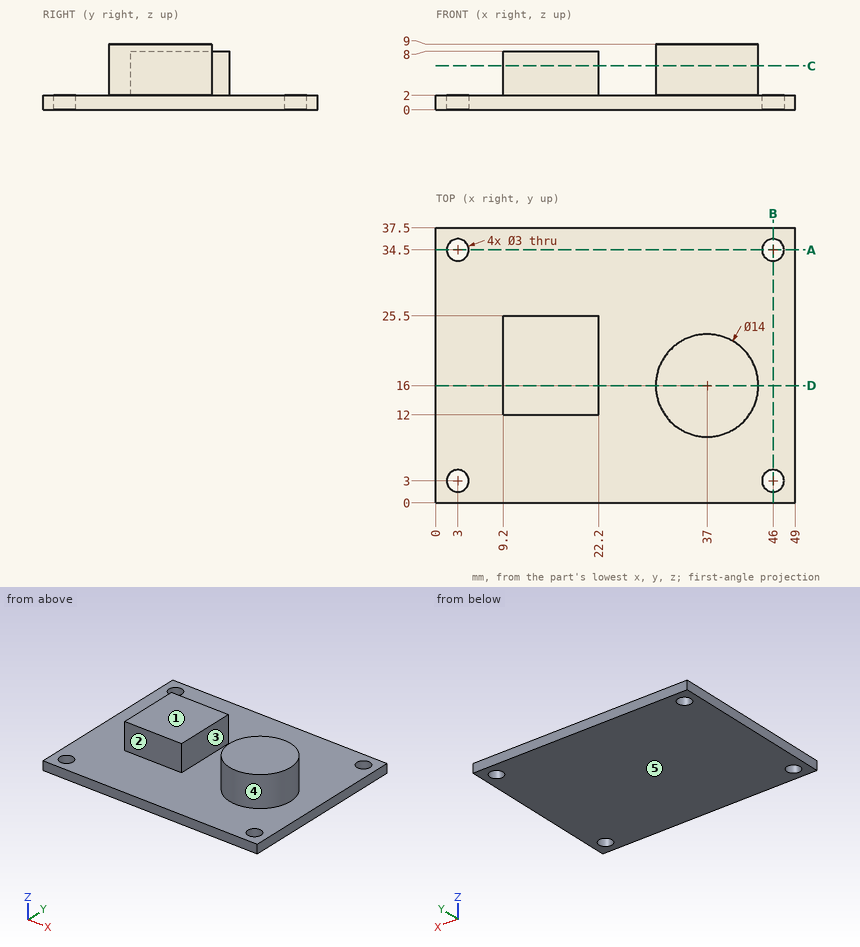
Can you work these out from the drawing? Everything is in mm from the part's minimum corner. A direction names the side the tool comes from. Coordinates: 2 decimals unless noted, no trailing zeros. Loops run counter-clockwise (first coordinate to the right, second up) from the corner with the lowest first, then second, coordinate; pieces in that order, holes last. Notation, with made-up numbers: M 7.5,14.25 L 60.5,14.25 A14 ccw 60.5,39.25 Z; hole C 2,71 d7. An arc over 180 degrees is marked long. Put each result on its own line as item: value. Start each with the question number.
(1) Thinking about a two-plate mould opening in X: for the marked faces 4 and 5, which applies, pulls with the +X half, pulls with the -X half, needs draft (parallel to the pull), parting line crosses it, or undercut?
(2) Will these pins go through, and if not, where does the flat tip stop? P1, Ø1.5, axis at x = 42.5, y = 10, coming from the +Z side; P2, Ø19, axis at x = 17, y = 16.5, coming from the +Z side; P3, Ø2, axis at y = 13.5, z = 3.5, coming from the +X side; P4, Ø1.8, axis at x = 3, y = 3, coming from the -Z side.
(3) For the marked faces 1, 2 and 3, which set-ups out of +Z, -Z, +X, -X, +Y, -Y let a thin tool reach every point of the face, with its end or its side?
(4) Suppose I cut it at C-C on z = 6. Please give me the cut outline in (x, y), then the cut area to 3 significant figures.
(5) Suppose I cut it at A-A on y = 34.5. Please give me the cut outline in (x, z), then the cut area to 3 significant figures.
(6) I need wall thicknesses on line 1 (Y direction, x = 46, z = 1.3); line 2 (Z direction, x = 33.5, y = 5); line 3 (Z direction, x = 12, y = 19.5). Which ranges of each line are inside material? Lowest first, please. Write a range as from..to.
(7) Suppose I cut it at D-D on y = 16. Please give me the cut outline in (x, z), then the cut area to 3 significant figures.
(8) Suppose I cut it at B-B on x = 46. Please give me the cut outline in (y, z), then the cut area to 3 significant figures.
Solutions:
1. face 4: undercut
1. face 5: needs draft
2. P1: stops at z = 2
2. P2: stops at z = 8
2. P3: stops at x = 43.84
2. P4: passes through
3. face 1: +Z, -X, +Y, -Y
3. face 2: +Z, -X, -Y
3. face 3: +Z, +Y, -Y
4. outline: M 9.2,12 L 22.2,12 L 22.2,25.5 L 9.2,25.5 Z; C 37,16 d14
4. area: 329 mm2
5. outline: M 0,0 L 1.5,0 L 1.5,2 L 0,2 Z; M 4.5,0 L 44.5,0 L 44.5,2 L 4.5,2 Z; M 47.5,0 L 49,0 L 49,2 L 47.5,2 Z
5. area: 86.0 mm2
6. line 1: y = 0..1.5, 4.5..33, 36..37.5
6. line 2: z = 0..2
6. line 3: z = 0..8
7. outline: M 0,0 L 49,0 L 49,2 L 44,2 L 44,9 L 30,9 L 30,2 L 22.2,2 L 22.2,8 L 9.2,8 L 9.2,2 L 0,2 Z
7. area: 274 mm2
8. outline: M 0,0 L 1.5,0 L 1.5,2 L 0,2 Z; M 4.5,0 L 33,0 L 33,2 L 4.5,2 Z; M 36,0 L 37.5,0 L 37.5,2 L 36,2 Z
8. area: 63.0 mm2
